Autodesk Inventor part; units mm, degrees
ref_plane "YZ Plane" through (0, 0, 0) normal (1, 0, 0) x (0, 1, 0)
ref_plane "XZ Plane" through (0, 0, 0) normal (0, 1, 0) x (-1, 0, 0)
ref_plane "XY Plane" through (0, 0, 0) normal (0, 0, 1) x (1, 0, 0)
sketch "Sketch1" plane through (0, 0, 0) normal (0, 0, 1) x (1, 0, 0)
  line L0 (-12.1, 6.05) -> (12.1, 6.05)
  line L1 (12.1, 6.05) -> (12.1, -6.05)
  line L2 (12.1, -6.05) -> (-12.1, -6.05)
  line L3 (-12.1, -6.05) -> (-12.1, 6.05)
  line L4 (-12.1, 6.05) -> (12.1, -6.05) construction
  line L5 (12.1, 6.05) -> (-12.1, -6.05) construction
  line L6 (-17.5, 12.5) -> (17.5, 12.5)
  line L7 (17.5, 12.5) -> (17.5, -12.5)
  line L8 (17.5, -12.5) -> (-17.5, -12.5)
  line L9 (-17.5, 12.5) -> (17.5, -12.5) construction
  line L10 (17.5, 12.5) -> (-17.5, -12.5) construction
  arc A0 (-43.9311, 7.3622) -> (-43.9311, -7.3622) centre (-42.5, 0) ccw
  line L11 (-17.5, 12.5) -> (-43.9311, 7.3622)
  line L12 (-17.5, -12.5) -> (-43.9311, -7.3622)
  point P0 (0, 0)
  point P1 (17.5, 0)
  dimension "d0" = 24.2
  dimension "d1" = 12.1
  dimension "d2" = 35
  dimension "d3" = 25
  dimension "d4" = 15
  dimension "d5" = 60
extrude "Extrusion1" add sketch "Sketch1" along normal blind 10
fillet "Fillet1" radius 4 2 edges at (17.5, 12.5, 5) (17.5, -12.5, 5)
sketch "Sketch2" plane through (0, 0, 10) normal (0, 0, 1) x (1, 0, 0)
  line L0 (12.1, 6.05) -> (12.1, -6.05)
  line L1 (-12.1, -6.05) -> (-12.1, 6.05)
  point P0 (0, 0)
  point P1 (14.3, 0)
  point P2 (-14.3, 0)
  dimension "d16" = 2.2
  dimension "d17" = 2.2
hole "Hole1" at (14.3, 0, 10) at (-14.3, 0, 10) direction (0, 0, -1) diameter 2.1 depth 8 tip angle 118
sketch "Sketch3" plane through (0, 0, 10) normal (0, 0, 1) x (1, 0, 0)
  line L0 (-18.5, 6) -> (-42.5, 3.5)
  line L1 (-18.5, -6) -> (-42.5, -3.5)
  line L2 (-42.5, -3.5) -> (-42.5, 3.5)
  line L3 (-42.5, 0) -> (-11.6221, -28.1421) construction
  line L4 (-30.5, 4.75) -> (-30.5, -4.75) construction
  arc A0 (-43.9311, 7.3622) -> (-43.9311, -7.3622) centre (-42.5, 0) ccw construction
  line L5 (-12.1, -6.05) -> (-12.1, 6.05)
  line L6 (-18.5, 6) -> (-18.5, -6)
  line L7 (-24.035, 5.4234) -> (-30.8838, -4.71)
  line L8 (-30.5, 4.75) -> (-36.4984, -4.1252)
  point P0 (0, 0)
  point P1 (-12.1, 0)
  point P2 (-12.1, 0)
  dimension "d27" = 7
  dimension "d31" = 24
  dimension "d32" = 6.5
  dimension "d33" = 12
  dimension "d34" = 50
  dimension "d35" = 50
extrude "Extrusion2" cut sketch "Sketch3" against normal blind 10
extrude "Extrusion3" add sketch "Sketch3" against normal blind 10 contours L7 L1 L8 L0
sketch "Sketch4" plane through (0, 0, 10) normal (0, 0, 1) x (1, 0, 0)
  arc A0 (-43.9311, 7.3622) -> (-43.9311, -7.3622) centre (-42.5, 0) ccw
  arc A1 (-47.7155, 7.1436) -> (-47.7155, -7.1436) centre (-50, 0) ccw
  line L0 (-17.5, 12.5) -> (-43.9311, 7.3622)
  arc A2 (-47.7155, 7.1436) -> (-30.7155, 9.9311) centre (-141.1455, 630.1772) ccw
  line L1 (-43.9311, -7.3622) -> (-17.5, -12.5)
  arc A3 (-30.7155, -9.9311) -> (-47.7155, -7.1436) centre (-141.1455, -630.1772) ccw
  line L2 (-18.5, 6) -> (-18.5, -6)
  point P0 (0, 0)
  point P1 (-18.5, 0)
  point P2 (-50, 0)
  dimension "d38" = 7.5
  dimension "d39" = 630
  dimension "d40" = 17
extrude "Extrusion4" add sketch "Sketch4" against normal blind 10
properties part number "pata_inferior_v3"
Geometry check sheet. Reference: the model listing, model coordinates, mm. A direction names the side the tool comes from. Coordinates: 2 decimals unless noted, no trailing zeros. Order: outer loops, then holes, each group sorted by start corner. A loop starts at its lowest first (then second) coordinate and runs counter-clockwise, first axis right, second up. Notation, with made-up numbers: (32.5, -4) - (74.5, -4) arc R12 cw to (74.5, 9) - close; hole circle Ø1 at (3.5, 6). An arc over 180 degrees is marked (long way). Answer in a Markdown table with one row per item. Add a question column.
1. Access from +Z, -Z, +X, -X, +Y, -Y to the whole of each face (thin tool, end or side, straight path). Record for faces 1 (the face through (-33.46, 0.37, 5.07)), 2 (the face through (-15.19, -0.56, 5.94)), 3 (the face through (16.359, 11.297, 5.07)).
2. Material ranges on L1, parallel to Y at x = -14.3, z = 8.25; L2, parallel to Y at x = -11.5, z = 8; L3, parallel to X at y = -3.25, z = 0.5, recorded low to high. Write a range as [from, to].
3. Draft check along Y on faces 4 (the face through (-2, 12.5, 5)), 5 (the face through (16.297, -11.359, 5.07)), 6 (the face through (-18.5, 0, 5)). Enter one of: +Y half, -Y half, draft (parallel to the pull), parting line (faces both ways), or undercut.
4. Section check A-A (z = 2.75). Give the number of separate pieces and of enclosed holes in the cut face, plus the area to 3 significant figures.
5. Section check B-B (x = -50). Enter the section's corners in (y, z), plus the area to 3 significant figures.
6. Gauge pin test, flat ends, axial feed: pin 1 Ø3 at (x, z) = (-45.5, 6.5) entering from -Y; pin 2 Ø1.7 at (x, y) = (14.3, 0) entering from +Z; pin 3 Ø3 at (y, z) = (-2.5, 5.5) entering from -X. Record the tip position at first contact, or that the pin passes through.
Data:
| question | item | result |
|---|---|---|
| 1 | face 1 | +Z, -Z |
| 1 | face 2 | +Z |
| 1 | face 3 | +Z, -Z, +X, +Y |
| 2 | L1 | y = [-12.5, -1.05], [1.05, 12.5] |
| 2 | L2 | y = [-12.5, -6.05], [6.05, 12.5] |
| 2 | L3 | x = [-56.76, -42.5], [-35.91, -29.9], [-18.5, -12.1], [12.1, 17.5] |
| 3 | face 4 | +Y half |
| 3 | face 5 | -Y half |
| 3 | face 6 | undercut |
| 4 | separate pieces | 1 |
| 4 | enclosed holes | 5 |
| 4 | area | 1,100 mm² |
| 5 | outline | (-7.5, 0) - (7.5, 0) - (7.5, 10) - (-7.5, 10) - close |
| 5 | area | 150 mm² |
| 6 | pin 1 | stops at y = -7.71 |
| 6 | pin 2 | stops at z = 1.88 |
| 6 | pin 3 | stops at x = -57.43 |
